Autodesk Inventor part; units mm, degrees
ref_plane "YZ Plane" through (0, 0, 0) normal (1, 0, 0) x (0, 1, 0)
ref_plane "XZ Plane" through (0, 0, 0) normal (0, 1, 0) x (-1, 0, 0)
ref_plane "XY Plane" through (0, 0, 0) normal (0, 0, 1) x (1, 0, 0)
sketch "Sketch1" plane through (0, 0, 0) normal (0, 1, 0) x (-1, 0, 0)
  line L0 (-24.4733, 28.5935) -> (-24.4733, -206.3565)
  line L1 (-24.4733, -206.3565) -> (118.5711, -106.1957)
  line L2 (-24.4733, -206.3565) -> (150.1517, -206.3565) construction
  line L3 (118.5711, -106.1957) -> (118.5711, -42.6957)
  line L4 (118.5711, -42.6957) -> (77.4122, 28.5935)
  line L5 (-24.4733, 28.5935) -> (77.4122, 28.5935)
  point P0 (0, 0)
  dimension "d0" = 234.95
  dimension "d1" = 174.625
  dimension "d2" = 35
  dimension "d3" = 63.5
  dimension "d4" = 150
extrude "Extrusion1" add sketch "Sketch1" along normal blind 3.175
sketch "Sketch2" plane through (0, 3.175, 0) normal (0, 1, 0) x (1, 0, 0)
  line L0 (-77.4122, -28.5935) -> (24.4733, -28.5935)
  line L1 (24.4733, -28.5935) -> (24.4733, 206.3565)
  line L2 (21.2983, 88.8815) -> (21.2983, 107.9315)
  line L3 (21.2983, 107.9315) -> (24.4733, 107.9315)
  line L4 (21.2983, 88.8815) -> (21.2983, 69.8315)
  line L5 (21.2983, 69.8315) -> (24.4733, 69.8315)
  point P0 (0, 0)
  dimension "d8" = 19.05
  dimension "d9" = 19.05
extrude "Extrusion2" add sketch "Sketch2" along normal blind 79.2734
sketch "Sketch3" plane through (24.4733, 0, 28.5935) normal (1, 0, 0) x (0, 0, -1)
  line L0 (136.525, 82.4484) -> (117.475, 82.4484)
  line L1 (117.475, 82.4484) -> (117.475, 63.3984)
  line L2 (117.475, 63.3984) -> (136.525, 63.3984)
  line L3 (136.525, 63.3984) -> (136.525, 82.4484)
  point P0 (28.5935, 0)
  dimension "d12" = 19.05
  dimension "d13" = 19.05
hole "Hole1" at (24.4733, 63.3984, -88.8815) direction (-1, 0, 0) diameter 8.3312 end through all
sketch "Sketch4" plane through (0, 3.175, 0) normal (0, 1, 0) x (1, 0, 0)
  line L0 (-102.9662, 117.1224) -> (-118.5711, 106.1957)
  line L1 (-118.5711, 87.1457) -> (-118.5711, 106.1957)
  line L2 (-124.1966, 109.1242) -> (-108.5917, 120.0508)
  line L3 (-124.1966, 109.1242) -> (-124.1966, 90.0742)
  line L4 (-102.9662, 117.1224) -> (-108.5917, 120.0508)
  line L5 (-118.5711, 87.1457) -> (-124.1966, 90.0742)
  point P0 (0, 0)
  dimension "d21" = 19.05
  dimension "d23" = 19.05
extrude "Extrusion3" add sketch "Sketch4" against normal blind 3.175
sketch "Sketch5" plane through (0, 3.175, 0) normal (0, 1, 0) x (1, 0, 0)
  line L0 (-108.5917, 120.0508) -> (-102.9662, 117.1224)
  line L1 (-124.1966, 109.1242) -> (-108.5917, 120.0508)
  line L2 (-124.1966, 90.0742) -> (-124.1966, 109.1242)
  line L3 (-118.5711, 87.1457) -> (-124.1966, 90.0742)
  line L4 (-124.1966, 90.0742) -> (-124.1966, 109.1242)
  line L5 (-124.1966, 109.1242) -> (-108.5917, 120.0508)
  line L6 (-108.5917, 120.0508) -> (-105.7755, 118.5848)
  line L7 (-105.7755, 118.5848) -> (-121.3838, 107.6557)
  line L8 (-121.3838, 107.6557) -> (-121.3838, 88.61)
  line L9 (-121.3838, 88.61) -> (-124.1966, 90.0742)
  point P0 (0, 0)
  dimension "d28" = 3.175
extrude "Extrusion4" add sketch "Sketch5" along normal blind 12.7
sketch "Sketch6" plane through (-108.5917, 0, -120.0508) normal (-0.5735764, 0, -0.819152) x (-0.819152, 0, 0.5735764)
  line L0 (19.05, 15.875) -> (19.05, 0)
  line L1 (0, 15.875) -> (19.05, 15.875)
  line L2 (9.525, 15.875) -> (9.525, 9.525)
  point P0 (-20.0948, 0)
  dimension "d31" = 6.35
hole "Hole2" at (-116.3942, 9.525, -114.5875) direction (0.5735764, 0, 0.819152) diameter 6.35 end through all
sketch "Sketch7" plane through (-124.1966, 0, -109.1242) normal (-1, 0, 0) x (0, 0, 1)
  line L0 (0, 15.875) -> (19.05, 15.875)
  line L1 (9.525, 15.875) -> (9.525, 9.525)
  point P0 (109.1242, 0)
  dimension "d39" = 6.35
hole "Hole3" at (-124.1966, 9.525, -99.5992) direction (1, 0, 0) diameter 6.35 depth 25.4 tip angle 118
sketch "Sketch8" plane through (21.2983, 3.175, -107.9315) normal (-1, 0, 0) x (0, 0, 1)
  line L0 (38.1, 0) -> (0, 0)
  line L1 (38.1, 0) -> (38.1, 79.2734)
  line L2 (0, 0) -> (0, 79.2734)
  line L3 (0, 41.1734) -> (38.1, 41.1734)
  line L4 (38.1, 41.1734) -> (38.1, 0)
  line L5 (38.1, 0) -> (0, 0)
  line L6 (0, 0) -> (0, 41.1734)
  point P0 (107.9315, -3.175)
  dimension "d47" = 38.1
extrude "Extrusion5" add sketch "Sketch8" along normal blind 25.4
sketch "Sketch9" plane through (21.2983, 82.4484, -69.8315) normal (0, 0, 1) x (1, 0, 0)
  line L0 (-25.4, -38.1) -> (3.175, -38.1)
  line L1 (3.175, -38.1) -> (3.175, -79.2734)
  line L2 (3.175, -79.2734) -> (-25.4, -79.2734)
  line L3 (-25.4, -79.2734) -> (-25.4, -38.1)
  point P0 (-21.2983, -82.4484)
extrude "Extrusion6" add sketch "Sketch9" along normal blind 25.4
sketch "Sketch13" plane through (24.4733, 0, 28.5935) normal (1, 0, 0) x (0, 0, -1)
  line L0 (98.425, 44.3484) -> (98.425, 82.4484)
  line L1 (147.5486, 3.175) -> (136.525, 44.3484)
  line L2 (147.5486, 3.175) -> (161.925, 3.175)
  line L3 (136.525, 44.3484) -> (161.925, 44.3484)
  line L4 (161.925, 44.3484) -> (161.925, 3.175)
  point P0 (28.5935, 0)
split_face "Split3"
sketch "Sketch14" plane through (24.4733, 0, 28.5935) normal (1, 0, 0) x (0, 0, -1)
  line L0 (161.925, 3.175) -> (234.95, 3.175)
  line L1 (136.525, 3.175) -> (147.5486, 3.175)
  line L2 (136.525, 44.3484) -> (136.525, 3.175)
  line L3 (136.525, 3.175) -> (147.5486, 3.175)
  line L4 (147.5486, 3.175) -> (136.525, 44.3484)
  point P0 (28.5935, 0)
  dimension "d73" = 11.0236
extrude "Extrusion8" add sketch "Sketch14" against normal blind 19.05
sketch "Sketch15" plane through (21.2983, 82.4484, -44.4315) normal (0, 0, 1) x (1, 0, 0)
  line L0 (0, -38.1) -> (-11.1125, -79.2734)
  line L1 (-11.1125, -79.2734) -> (-25.4, -79.2734)
  line L2 (-25.4, -79.2734) -> (-25.4, -38.1)
  line L3 (-25.4, -38.1) -> (0, -38.1)
  point P0 (-21.2983, -82.4484)
split body "Split4" sketch "Sketch15" result one side removed curves L0 L1 L2 L3 removed pieces at (13.4073, 17.0298, -77.7394)
sketch "Sketch16" plane through (24.4733, 0, 28.5935) normal (1, 0, 0) x (0, 0, -1)
  line L0 (87.4014, 3.175) -> (98.425, 44.3484)
  line L1 (87.4014, 3.175) -> (73.025, 3.175)
  line L2 (73.025, 3.175) -> (73.025, 44.3484)
  line L3 (73.025, 44.3484) -> (98.425, 44.3484)
  point P0 (28.5935, 0)
split body "Split5" sketch "Sketch16" result one side removed curves L3 L0 L1 L2 removed pieces at (18.0769, 30.4936, -57.6903)
properties part number "Right Chest"
Check sheet for the modelled part. Datum: model origin and axes. Units: mm. A direction names the side the tool comes from. Give positions to 0.01 mm unless a question says otherwise; leave off trailing zeros. Write each loop counter-clockwise with the first axis right and the second up, starting at its lowest first coordinate (ties: lowest second). Pieces come first, ordered by that corner, then holes. Notation, with made-up numbers: M 17,88.5 L 33,88.5 A19 ccw 33,113.5 Z; hole C -14,42 d4. An arc over 180 degrees is marked long. Use one line per item in the form item = value.
(1) Section check B-B on y = 50. Record the boundary of the cut face in (x, z), plus the area to 3 significant figures.
Answer block:
outline = M 21.3,-107.93 L 24.47,-107.93 L 24.47,-69.83 L 21.3,-69.83 Z
area = 121 mm2
(2) Material ranges on line 1 along Y through (x, z) = (-25, -54) (3 decimals); line 2 along X through (y, z) = (56, -90.5); line 3 along X through (y, z) = (10.5, -94), recorded low to high.
Answer block:
line_1 = 0 to 3.175
line_2 = 21.3 to 24.47
line_3 = -124.2 to -121.38, 12.16 to 24.47
(3) Section check C-C on x = -32. Record the boundary of the cut face in (y, z) (1 decimal), plus the area to 3 significant figures.
Answer block:
outline = M 0,-166.8 L 3.2,-166.8 L 3.2,28.6 L 0,28.6 Z
area = 620 mm2
(4) Tool access check on faces 4 (the cylindrical face through (-122.77, 9.39, -102.77)), 5 (the flat face through (-111.74, 9.44, -114.41)), 6 (the flat face through (15.82, 24.05, -89.3)). Record the directions out of +Z, -Z, +X, -X, +Y, -Y that give a thin tool (end or side, any length) a straight path to the whole face; none if there is none.
Answer block:
face_4 = -X
face_5 = +Z, +Y
face_6 = +Z, -Z, +Y
(5) Depth check by flat-ended pin: P1, Ø19, axis at y = 69, z = -90, coming from the -X side; P2, Ø2.5, axis at x = 23.5, y = 63, coming from the +Z side; P3, Ø12, axis at y = 10.5, z = -69, coming from the -X side. Enter the tip coordinate at first touch or a pass-through.
Answer block:
P1 = 21.3
P2 = -69.83
P3 = 10.54
(6) Section check A-A on z = -78.5. Record the boundary of the cut face in (x, y) (3 decimals), plus the area to 3 significant figures.
Answer block:
outline = M -118.571,0 L 24.473,0 L 24.473,82.448 L 21.298,82.448 L 21.298,44.348 L 10.186,3.175 L -118.571,3.175 Z
area = 935 mm2
(7) Draft check along X on faces 1 (the flat face through (-122, 15.875, -107)), 2 (the flat face through (-98.28, 1.57, -7.55)), 3 (the flat face through (-121.384, 9, -96)). Enter one of: pulls with the +X half, pulls with the -X half, needs draft (parallel to the pull), parting line crosses it, or undercut.
Answer block:
face_1 = needs draft
face_2 = pulls with the -X half
face_3 = undercut
